Source: CAD feature listing. Evaluate the final solid. Frame: model axes, mm. Face numbers are marked on the shaded views. A direction names the side the tool comes from. Coordinates: 2 decimals unless noted, no trailing zeros. Write each loop counter-clockwise with the first axis right and the second up, starting at its lowest first coordinate (ties: lowest second). Pieces come first, ordered by that corner, then holes. Notation, with made-up numbers: M -2.75,50 L 33.25,50 A22 cw 33.25,85 Z; hole C 1.25,-36.5 d11. An arc over 180 degrees is marked long. Answer as CSV lines item,"result". Start each with the question number.
1. Line query: probe 1 along Z at (x, y) = (-6.3, 0); probe 2 along Z at (x, y) = (7.25, 0). Output: solid intervals per line, ascending. Write a range as [from, to].
2. Section C-C on z = -54. Return the cut outline in (x, y), plus the area to 3 significant figures.
3. Contact query for flat-ended pins moving along their axis: pin 1 Ø8.5 at (y, z) = (-2, -1.5) entering from -X; pin 2 Ø2.5 at (x, z) = (-5, -2.5) entering from -Y; pin 3 Ø10 at (y, z) = (-32.5, 46.5) entering from -X. Output: stop coordinate, or through.
4. Section A-A on x = 9.5. Return the cut outline in (y, z) (1 decimal).
5. Section B-B on y = -43. Return the cut outline in (x, z), plus the area to 3 significant figures.
6. Reachability of the marked faces 1 and 2 from +Z, -Z, +X, -X, +Y, -Y: full face, straight path, thin tool, end or side. Return the list, or none.
7. Section D-D on x = 50. Return the cut outline in (y, z).
```python
from build123d import *

# Parameters (mm, degrees)
SKETCH1_W               = 81
SKETCH1_H               = 12.5
SKETCH2_W               = 31.25
SKETCH2_H               = 62.5
CUT_EXTRUDE1_DEPTH      = 25
CUT_EXTRUDE1_DEPTH_BACK = 25


with BuildPart() as part:
    # Sketch1 → Revolve1 (revolve)
    with BuildSketch(Plane.XY):
        with Locations((29.5, 6.25)):
            Rectangle(SKETCH1_W, SKETCH1_H)
    revolve(axis=Axis((70, 0, 0), (-1, 0, 0)))

    # Sketch2 → Revolve2 (revolve)
    with BuildSketch(Plane.XY):
        with Locations((54.375, 31.25)):
            Rectangle(SKETCH2_W, SKETCH2_H)
    revolve(axis=Axis((70, 0, 0), (-1, 0, 0)))

    # Sketch3 → Cut-Extrude1 (cut, two sides)
    with BuildSketch(Plane.XY) as cut_extrude1_sk:
        Polygon((-67, -28), (8.103629711, -28), (-2, -10.5), (-11, -10.5), (-11, -15.5), (-56, -15.5), (-56, 15.5), (-11, 15.5), (-11, 10.5), (-2, 10.5), (8.103629711, 28), (-67, 28), align=None)
    extrude(amount=CUT_EXTRUDE1_DEPTH, mode=Mode.SUBTRACT)
    extrude(cut_extrude1_sk.sketch, amount=-CUT_EXTRUDE1_DEPTH_BACK, mode=Mode.SUBTRACT)

    # Sketch4 → Cut-Revolve1 (revolve, cut)
    with BuildSketch(Plane.XY):
        Polygon((-11, 0), (-11, 9.5), (-10, 8.5), (-4, 8.5), (-4, 8), (-2.9175, 6.9175), (20.5, 6.9175), (24.493820487, 0), align=None)
    revolve(axis=Axis((24.493820487, 0, 0), (-1, 0, 0)), mode=Mode.SUBTRACT)


solid = part.part
```
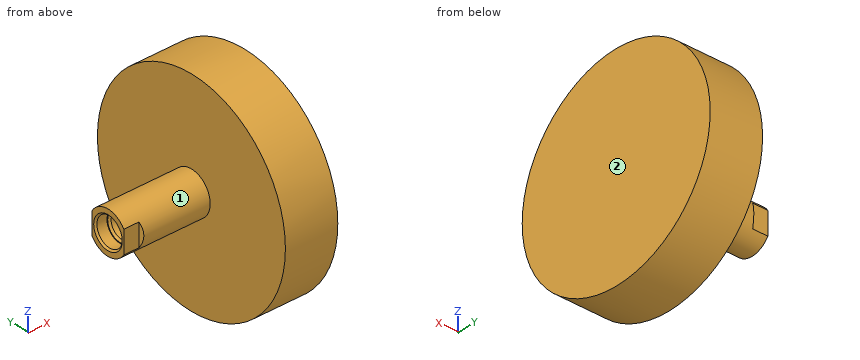
Values:
1,probe 1,"[-12.5, -8.5], [8.5, 12.5]"
1,probe 2,"[-12.5, -6.92], [6.92, 12.5]"
2,outline,"M 38.75,-31.47 L 70,-31.47 L 70,31.47 L 38.75,31.47 Z"
2,area,"1,970 mm²"
3,pin 1,"x = 20.6"
3,pin 2,"y = -10.5"
3,pin 3,"x = 38.75"
4,outline,"C 0,0 d25; hole C 0,0 d13.8"
5,outline,"M 38.75,-45.36 L 70,-45.36 L 70,45.36 L 38.75,45.36 Z"
5,area,"2,830 mm²"
6,face 1,"-X"
6,face 2,"+Z, -Z, +X, +Y, -Y"
7,outline,"C 0,0 d125"
